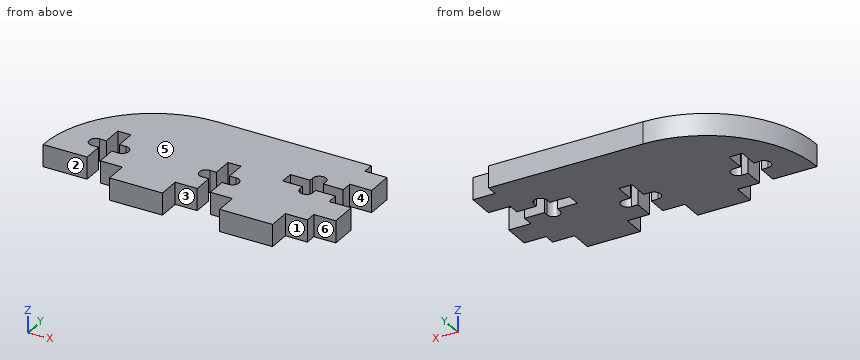
from build123d import *

# Parameters (mm, degrees)
BOSS_EXTRUDE1_DEPTH = 5


with BuildPart() as part:
    # Sketch1 → Boss-Extrude1 (new body)
    with BuildSketch(Plane.XY):
        with BuildLine():
            Line((23.963951988, -5.840885969), (18.963951988, -5.840885969))
            Line((18.963951988, -5.840885969), (18.963951988, -10.840885969))
            Line((18.963951988, -10.840885969), (6.963951988, -10.840885969))
            Line((6.963951988, -10.840885969), (6.963951988, -5.840885969))
            Line((6.963951988, -5.840885969), (1.963951988, -5.840885969))
            Line((1.963951988, -5.840885969), (1.963951988, -1.340885969))
            Line((1.963951988, -1.340885969), (3.463951988, -1.340885969))
            ThreePointArc((3.463951988, -1.340885969), (4.963951988, 0.159114031), (3.463951988, 1.659114031))
            Line((3.463951988, 1.659114031), (1.963951988, 1.659114031))
            Line((1.963951988, 1.659114031), (1.963951988, 6.159114031))
            Line((1.963951988, 6.159114031), (-1.036048012, 6.159114031))
            Line((-1.036048012, 6.159114031), (-1.036048012, 1.659114031))
            Line((-1.036048012, 1.659114031), (-2.536048012, 1.659114031))
            ThreePointArc((-2.536048012, 1.659114031), (-4.036048012, 0.159114031), (-2.536048012, -1.340885969))
            Line((-2.536048012, -1.340885969), (-1.036048012, -1.340885969))
            Line((-1.036048012, -1.340885969), (-1.036048012, -5.840885969))
            Line((-1.036048012, -5.840885969), (-6.036048012, -5.840885969))
            Line((-6.036048012, -5.840885969), (-6.036048012, -10.840885969))
            Line((-6.036048012, -10.840885969), (-18.036048012, -10.840885969))
            Line((-18.036048012, -10.840885969), (-18.036048012, -5.840885969))
            Line((-18.036048012, -5.840885969), (-23.036048012, -5.840885969))
            Line((-23.036048012, -5.840885969), (-23.036048012, -1.340885969))
            Line((-23.036048012, -1.340885969), (-21.536048012, -1.340885969))
            ThreePointArc((-21.536048012, -1.340885969), (-20.036048012, 0.159114031), (-21.536048012, 1.659114031))
            Line((-21.536048012, 1.659114031), (-23.036048012, 1.659114031))
            Line((-23.036048012, 1.659114031), (-23.036048012, 6.159114031))
            Line((-23.036048012, 6.159114031), (-26.036048012, 6.159114031))
            Line((-26.036048012, 6.159114031), (-26.036048012, 1.659114031))
            Line((-26.036048012, 1.659114031), (-27.536048012, 1.659114031))
            ThreePointArc((-27.536048012, 1.659114031), (-29.036048012, 0.159114031), (-27.536048012, -1.340885969))
            Line((-27.536048012, -1.340885969), (-26.036048012, -1.340885969))
            Line((-26.036048012, -1.340885969), (-26.036048012, -5.840885969))
            Line((-26.036048012, -5.840885969), (-36.036048012, -5.840885969))
            ThreePointArc((-36.036048012, -5.840885969), (-28.713717542, 11.836783561), (-11.036048012, 19.159114031))
            Line((-11.036048012, 19.159114031), (23.963951988, 19.159114031))
            Line((23.963951988, 19.159114031), (23.963951988, 16.659114031))
            Line((23.963951988, 16.659114031), (28.963951988, 16.659114031))
            Line((28.963951988, 16.659114031), (28.963951988, 10.659114031))
            Line((28.963951988, 10.659114031), (23.963951988, 10.659114031))
            Line((23.963951988, 10.659114031), (23.963951988, 8.159114031))
            Line((23.963951988, 8.159114031), (19.463951988, 8.159114031))
            Line((19.463951988, 8.159114031), (19.463951988, 9.159114031))
            ThreePointArc((19.463951988, 9.159114031), (17.963951988, 10.659114031), (16.463951988, 9.159114031))
            Line((16.463951988, 9.159114031), (16.463951988, 8.159114031))
            Line((16.463951988, 8.159114031), (11.963951988, 8.159114031))
            Line((11.963951988, 8.159114031), (11.963951988, 5.159114031))
            Line((11.963951988, 5.159114031), (16.463951988, 5.159114031))
            Line((16.463951988, 5.159114031), (16.463951988, 4.159114031))
            ThreePointArc((16.463951988, 4.159114031), (17.963951988, 2.659114031), (19.463951988, 4.159114031))
            Line((19.463951988, 4.159114031), (19.463951988, 5.159114031))
            Line((19.463951988, 5.159114031), (23.963951988, 5.159114031))
            Line((23.963951988, 5.159114031), (23.963951988, 2.659114031))
            Line((23.963951988, 2.659114031), (28.963951988, 2.659114031))
            Line((28.963951988, 2.659114031), (28.963951988, -3.340885969))
            Line((28.963951988, -3.340885969), (23.963951988, -3.340885969))
            Line((23.963951988, -3.340885969), (23.963951988, -5.840885969))
        make_face()
    extrude(amount=BOSS_EXTRUDE1_DEPTH)


solid = part.part
The model under review builds one solid part; all positions refer to its coordinate system, in mm. Face numbers are marked on the shaded views. A direction names the side the tool comes from. Round coordinates to 2 decimals unless told otherwise and drop trailing zeros. Write each loop counter-clockwise with the first axis right and the second up, starting at its lowest first coordinate (ties: lowest second). Pieces come first, ordered by that corner, then holes. Notation, with made-up numbers: M 85,32.25 L 96,32.25 A21 ccw 96,43.25 Z; hole C 44.25,-1.75 d4. An arc over 180 degrees is marked long. Answer as CSV lines item,"result". Start each with the question number.
Q1. Consider section C-C, the plane y = 15. Give the boundary of the cut face in (x, z).
Q2. Clearance check with flat-ended pins moving along their axes: P1, Ø0.5, axis at x = -2, z = 2.5, coming from the -Y side; P2, Ø1.3, axis at y = -4.5, z = 3, coming from the +X side; P3, Ø1.5, axis at x = -24.5, z = 2.5, coming from the -Y side. State where each tip first meets the part, or that it passes through.
Q3. Tool access review of the marked faces 1, 2 and 3: name each direction out of +Z, -Z, +X, -X, +Y, -Y from which nothing blocks a thin tool from reaching the whole face with its end or side.
Q4. The part is to be moulded in two halves that separate along Y. For the marked faces 4, 5 and 6, say which applies: +Y half, -Y half, draft (parallel to the pull), parting line (faces both ways), or undercut.
Q5. Consider section A-A, the plane y = -6.5. Give the boundary of the cut face in (x, z), then the cut area to 3 significant figures.
Q6. Consider section B-B, the plane x = 0. Give the boundary of the cut face in (y, z), then the cut area to 3 significant figures.
Q7. Wall thickness on line 1 along X through (y, z) = (-5.5, 3.6); line 2 along Y through (x, z) = (-2.5, 4.25); line 3 along Y through (x, z) = (15, 1.55): over which ranges is each line inside the solid? List them lowest first.
Result set:
1,outline,"M -24.84,0 L 28.96,0 L 28.96,5 L -24.84,5 Z"
2,P1,"stops at y = -5.84"
2,P2,"stops at x = 23.96"
2,P3,"stops at y = 6.16"
3,face 1,"+Z, -Z, +X, -Y"
3,face 2,"+Z, -Z, -X, -Y"
3,face 3,"+Z, -Z, -Y"
4,face 4,"undercut"
4,face 5,"draft"
4,face 6,"-Y half"
5,outline,"M -18.04,0 L -6.04,0 L -6.04,5 L -18.04,5 Z; M 6.96,0 L 18.96,0 L 18.96,5 L 6.96,5 Z"
5,area,"120 mm²"
6,outline,"M 6.16,0 L 19.16,0 L 19.16,5 L 6.16,5 Z"
6,area,"65.0 mm²"
7,line 1,"x = -36.03 to -26.04, -23.04 to -1.04, 1.96 to 23.96"
7,line 2,"y = -5.84 to -1.34, 1.66 to 19.16"
7,line 3,"y = -10.84 to 5.16, 8.16 to 19.16"
